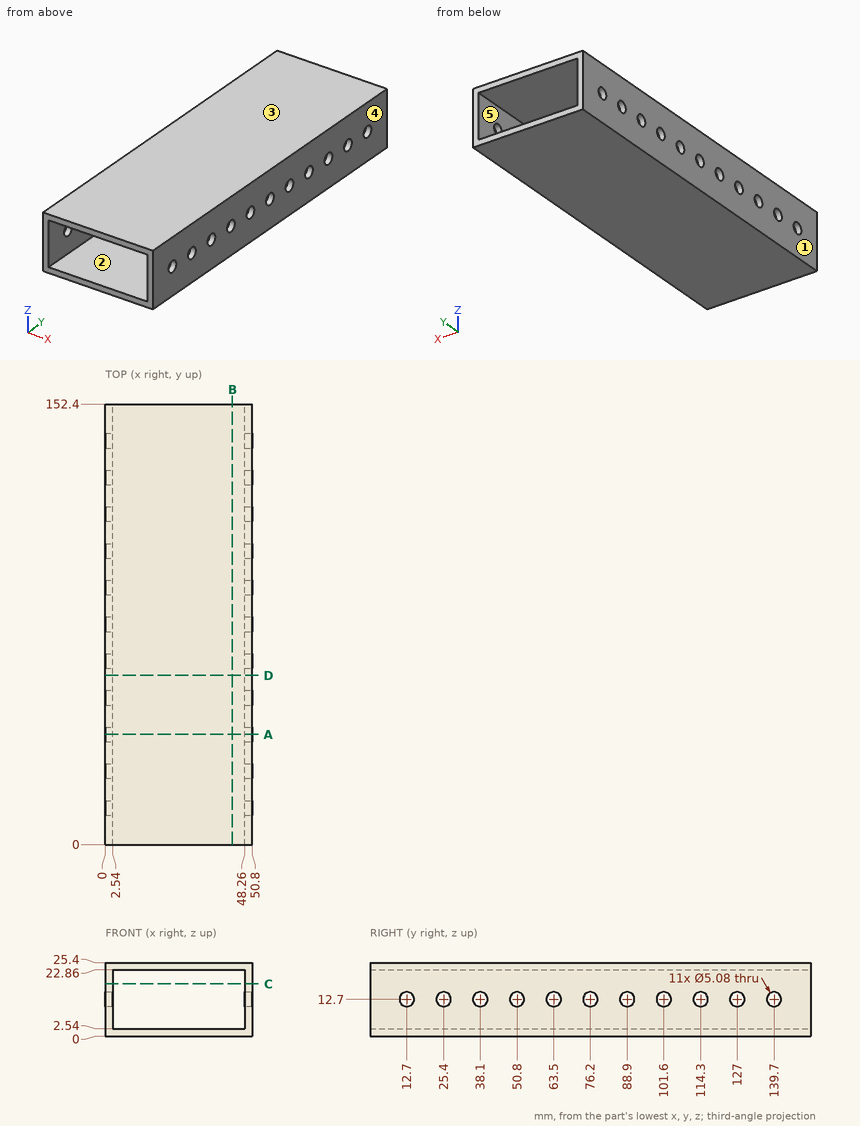
For this review, use the dimensioned drawing (mm, ordinates from the lowest corner) and the shaded views. A direction names the side the tool comes from. Give positions to 0.01 mm unless a question says otherwise; leave off trailing zeros. Write each loop counter-clockwise with the first axis right and the second up, starting at its lowest first coordinate (ties: lowest second). Pieces come first, ordered by that corner, then holes.
(1) The part is to be moulded in two halves that separate along X. For the marked faces 3, 4 and 5, say which applies: released by +X, released by -X, zero draft, split by the parting line, or undercut.
(2) Consider section A-A, the plane y = 38.1. Give the boundary of the cut face in (x, z).
(3) Consider section B-B, the plane x = 44. Give the boundary of the cut face in (y, z), and give its area (3 significant figures).
(4) To check wall thickness, follow L1, parallel to X at y = 79, z = 8.25; L2, parallel to Z at x = 36, y = 8.5; L3, parallel to Z at x = 1.1, y = 139.7. State the ranges of each line that lie inside material, in increasing order.
(5) Consider section D-D, the plane y = 58.5. Give the boundary of the cut face in (x, z), and give its area (3 significant figures).
(6) Consider section C-C, the plane z = 18. Give the boundary of the cut face in (x, y), and give its area (3 significant figures).
(7) For P1, Ø6.5, axis at y = 25.4, z = 12.7, coming from the -X side, flat-tipped, find the tip position at first contact; note if it passes through.
(8) Tool access review of the marked faces 1 and 2: name each direction out of +Z, -Z, +X, -X, +Y, -Y from which nothing blocks a thin tool from reaching the whole face with its end or side.
Returned:
1. face 3: zero draft
1. face 4: released by +X
1. face 5: undercut
2. outline: (0, 0) - (50.8, 0) - (50.8, 10.16) - (48.26, 10.16) - (48.26, 2.54) - (2.54, 2.54) - (2.54, 10.16) - (0, 10.16) - close; (0, 15.24) - (2.54, 15.24) - (2.54, 22.86) - (48.26, 22.86) - (48.26, 15.24) - (50.8, 15.24) - (50.8, 25.4) - (0, 25.4) - close
3. outline: (0, 0) - (152.4, 0) - (152.4, 2.54) - (0, 2.54) - close; (0, 22.86) - (152.4, 22.86) - (152.4, 25.4) - (0, 25.4) - close
3. area: 774 mm2
4. L1: x = 0 to 2.54, 48.26 to 50.8
4. L2: z = 0 to 2.54, 22.86 to 25.4
4. L3: z = 0 to 10.16, 15.24 to 25.4
5. outline: (0, 0) - (50.8, 0) - (50.8, 25.4) - (0, 25.4) - close; hole (2.54, 2.54) - (48.26, 2.54) - (48.26, 22.86) - (2.54, 22.86) - close
5. area: 361 mm2
6. outline: (0, 0) - (2.54, 0) - (2.54, 152.4) - (0, 152.4) - close; (48.26, 0) - (50.8, 0) - (50.8, 152.4) - (48.26, 152.4) - close
6. area: 774 mm2
7. P1: stops at x = 0
8. face 1: +Z, -Z, -X, +Y, -Y
8. face 2: +Y, -Y
